Could you check a few things on this model? Use its own coordinates, in mm. Face numbers are marked on the shaded views. A direction names the side the tool comes from. Coordinates: 2 decimals unless noted, no trailing zeros. Loops run counter-clockwise (first coordinate to the right, second up) from the corner with the lowest first, then second, coordinate; pieces in that order, holes last. Notation, with made-up numbers: (56, 46) -> (113, 46) arc R10 cw to (113, 55) -> close; hole circle Ø4 at (56.5, -23). An arc over 180 degrees is marked (long way). One line per question, with ' | ' between items.
Autodesk Inventor part; units mm, degrees
ref_plane "YZ Plane" through (0, 0, 0) normal (1, 0, 0) x (0, 1, 0)
ref_plane "XZ Plane" through (0, 0, 0) normal (0, 1, 0) x (-1, 0, 0)
ref_plane "XY Plane" through (0, 0, 0) normal (0, 0, 1) x (1, 0, 0)
sketch "Skizze1" plane through (0, 0, 0) normal (0, 0, 1) x (1, 0, 0)
  line L0 (11.5, 38) -> (-11.5, 38)
  line L1 (-11.5, 38) -> (-11.5, -38)
  line L2 (-11.5, -38) -> (11.5, -38)
  line L3 (11.5, -38) -> (11.5, 38)
  line L4 (11.5, 38) -> (-11.5, -38) construction
  line L5 (-11.5, 38) -> (11.5, -38) construction
  line L6 (-23, -50) -> (23, -50)
  line L7 (23, -50) -> (23, -38)
  line L8 (23, -38) -> (-23, -38)
  line L9 (-23, -38) -> (-23, -50)
  line L10 (-23, -50) -> (23, -38) construction
  line L11 (23, -50) -> (-23, -38) construction
  line L12 (-23, -38) -> (-11.5, -38)
  line L13 (-11.5, -38) -> (-11.5, -8)
  line L14 (-11.5, -8) -> (-23, -8)
  line L15 (-23, -8) -> (-23, -38)
  line L16 (23, -38) -> (11.5, -38)
  line L17 (11.5, -38) -> (11.5, -8)
  line L18 (11.5, -8) -> (23, -8)
  line L19 (23, -8) -> (23, -38)
  point P0 (0, 0)
  point P1 (0, -44)
  point P2 (0, -38)
  dimension "d0" = 23
  dimension "d1" = 76
  dimension "d2" = 12
  dimension "d3" = 30
  dimension "d4" = 30
  dimension "d5" = 46
extrude "Extrusion1" add sketch "Skizze1" along normal blind 10 contours L18 L19 L8 L3 | L1 L8 L15 L14 | L8 L7 L6 L9 L2
sketch "Skizze2" plane through (-11.5, -38, 0) normal (1, 0, 0) x (0, 0, -1)
  line L0 (0, 30) -> (0, -12)
  line L1 (0, -7.7211) -> (-0.5, -7.7211)
  line L2 (-0.5, -7.7211) -> (-2, -3.621)
  line L3 (-2, -3.621) -> (-2, 30)
  line L4 (-2, 30) -> (0, 30)
  line L5 (0, 0) -> (0, 30)
  point P0 (0, 38)
  point P1 (0, 5.0638)
  dimension "d8" = 0.5
  dimension "d15" = 2
extrude "Extrusion2" cut sketch "Skizze2" along normal blind 25 and the other way blind 2
sketch "Skizze3" plane through (-23, -50, 0) normal (-1, 0, 0) x (0, 0, 1)
  line L0 (0, 42) -> (0, 0)
  line L1 (0, 0) -> (10, 0)
  line L2 (10, 42) -> (10, 0)
  line L3 (0, 42) -> (10, 42)
  circle A0 centre (6.7241, 56.1881) radius 1.5
  point P0 (0, 50)
  dimension "d11" = 3
extrude "Extrusion3" cut sketch "Skizze3" against normal through all contours A0
fillet "Rundung1" radius 2 4 edges at (17.25, -8, 10) (-17.25, -8, 10) (-23, -50, 5) (23, -50, 5)
sketch "Skizze4" plane through (0, 0, 0) normal (0, 0, -1) x (-1, 0, 0)
  arc A0 (-23, -48) -> (-21, -50) centre (-21, -48) ccw
  line L0 (21, -50) -> (-21, -50)
  arc A1 (21, -50) -> (23, -48) centre (21, -48) ccw
  line L1 (23, -8) -> (23, -48)
  line L2 (13.5, -8) -> (23, -8)
  line L3 (13.5, -8) -> (13.5, -45.7211)
  line L4 (13.5, -45.7211) -> (-13.5, -45.7211)
  line L5 (-13.5, -45.7211) -> (-13.5, -8)
  line L6 (-23, -8) -> (-13.5, -8)
  line L7 (-23, -48) -> (-23, -8)
  line L8 (-25, -6) -> (-11.5, -6)
  line L9 (-11.5, -6) -> (-11.5, -43.7211)
  line L10 (-11.5, -43.7211) -> (11.5, -43.7211)
  line L11 (11.5, -43.7211) -> (11.5, -6)
  line L12 (11.5, -6) -> (25, -6)
  line L13 (25, -6) -> (25, -48)
  arc A2 (21, -52) -> (25, -48) centre (21, -48) ccw
  line L14 (21, -52) -> (-21, -52)
  arc A3 (-25, -48) -> (-21, -52) centre (-21, -48) ccw
  line L15 (-25, -48) -> (-25, -6)
  line L16 (-23, -8) -> (-25, -8)
  line L17 (23, -8) -> (25, -8)
  point P0 (0, 0)
  dimension "d18" = 2
extrude "Extrusion4" add sketch "Skizze4" against normal blind 2 contours A0 L0 A1 L1 L17 L13 A2 L14 A3 L15 L16 L7
sketch "Skizze5" plane through (0, 0, 10) normal (0, 0, 1) x (1, 0, 0)
  arc A0 (21, -50) -> (23, -48) centre (21, -48) ccw
  line L0 (23, -48) -> (23, -10)
  line L1 (11.5, -10) -> (23, -10)
  line L2 (11.5, -10) -> (11.5, -38)
  line L3 (11.5, -38) -> (-11.5, -38)
  line L4 (-11.5, -38) -> (-11.5, -10)
  line L5 (-23, -10) -> (-11.5, -10)
  line L6 (-23, -10) -> (-23, -48)
  arc A1 (-23, -48) -> (-21, -50) centre (-21, -48) ccw
  line L7 (-21, -50) -> (21, -50)
  line L8 (-17.1067, -44.1067) -> (-17.1067, -15.8933)
  line L9 (-17.1067, -15.8933) -> (-17.3933, -15.8933)
  line L10 (-17.3933, -15.8933) -> (-17.3933, -43.8933)
  line L11 (-17.3933, -43.8933) -> (17.3933, -43.8933)
  line L12 (17.3933, -43.8933) -> (17.3933, -15.8933)
  line L13 (17.3933, -15.8933) -> (17.1067, -15.8933)
  line L14 (17.1067, -15.8933) -> (17.1067, -44.1067)
  line L15 (17.1067, -44.1067) -> (-17.1067, -44.1067)
  point P0 (0, 0)
hole "Bohrung1" at (-17.1067, -44.1067, 10) at (17.1067, -44.1067, 10) at (17.1067, -15.8933, 10) at (-17.1067, -15.8933, 10) direction (0, 0, -1) diameter 2.8 depth 12 tip angle 118
properties part number "Anglerfish_coverslipclamp_top_short"
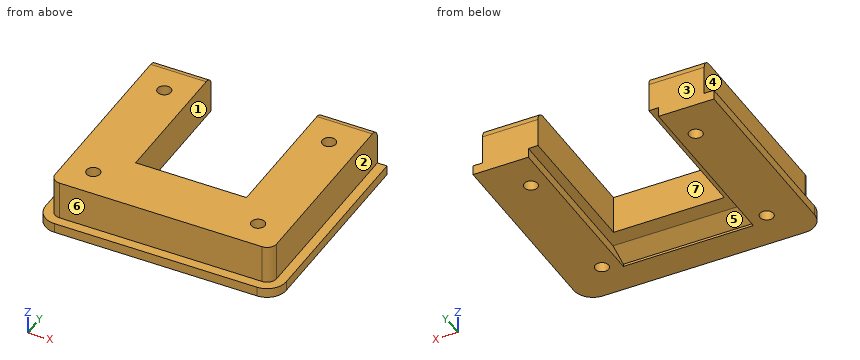
Q1. We'd pull the mould along X, two halves only. Please class the marked faces 1, 2, 3 and 4: released by +X, released by -X, zero draft, split by the parting line, or undercut.
Values follow:
face 1: undercut | face 2: released by +X | face 3: zero draft | face 4: released by -X
Q2. Please list where these lines run through material, in increasing order: L1, parallel to X at y = -12, z = 4; L2, parallel to X at y = -26, z = 1; L3, parallel to X at y = -16.5, z = 7.25. Write a range as [from, to].
Values follow:
L1: x = [-23, -11.5], [11.5, 23] | L2: x = [-25, -13.5], [13.5, 25] | L3: x = [-23, -18.37], [-15.84, -11.5], [11.5, 15.84], [18.37, 23]
Q3. Imagine slicing it at B-B on x = -8.5. Write out the boundary of the cut face in (y, z).
Values follow:
outline: (-52, 0) -> (-45.72, 0) -> (-45.72, 0.5) -> (-41.62, 2) -> (-38, 2) -> (-38, 10) -> (-50, 10) -> (-50, 2) -> (-52, 2) -> close
Q4. For the marked faces 5, 6 and 7, which set-ups out of +Z, -Z, +X, -X, +Y, -Y let a thin tool reach every point of the face, with its end or its side?
Values follow:
face 5: -Z, +Y | face 6: +Z, +X, -X, -Y | face 7: +Z, -Z, +Y
Q5. Imagine slicing it at C-C on z = 3. Write out the boundary of the cut face in (x, y).
Values follow:
outline: (-23, -48) arc R2 ccw to (-21, -50) -> (21, -50) arc R2 ccw to (23, -48) -> (23, -8) -> (11.5, -8) -> (11.5, -38) -> (-11.5, -38) -> (-11.5, -8) -> (-23, -8) -> close; hole circle Ø2.8 at (-17.11, -44.11); hole circle Ø2.8 at (-17.11, -15.89); hole circle Ø2.8 at (17.11, -44.11); hole circle Ø2.8 at (17.11, -15.89)
Q6. For pin 1 (6 mm diameter, centred on y = -43, z = 7, fed in from +X); pin 2 (6 mm diameter, centred on x = 2.5, z = 1, fed in from +Y); pin 3 (4 mm diameter, centred on x = 10.5, z = 6, fed in from -Y), each with a flat end and sliding along its axis, tell me the tip position at first contact or that it passes through.
Values follow:
pin 1: stops at x = 23 | pin 2: stops at y = -38 | pin 3: stops at y = -50
Q7. Imagine slicing it at D-D on x = -16.5. Write out the boundary of the cut face in (y, z).
Values follow:
outline: (-52, 0) -> (-45.37, 0) -> (-45.37, 10) -> (-50, 10) -> (-50, 2) -> (-52, 2) -> close; (-42.84, 0) -> (-17.16, 0) -> (-17.16, 10) -> (-42.84, 10) -> close; (-14.63, 0) -> (-8, 0) -> (-8, 8) arc R2 ccw to (-10, 10) -> (-14.63, 10) -> close
Q8. Imagine slicing it at A-A on y = -36.5. Write out the boundary of the cut face in (x, z), plus the area to 3 significant figures.
Values follow:
outline: (-25, 0) -> (-13.5, 0) -> (-13.5, 2) -> (-11.5, 2) -> (-11.5, 10) -> (-23, 10) -> (-23, 2) -> (-25, 2) -> close; (11.5, 2) -> (13.5, 2) -> (13.5, 0) -> (25, 0) -> (25, 2) -> (23, 2) -> (23, 10) -> (11.5, 10) -> close | area: 230 mm2
